Geometry check sheet. Reference: the model listing, model coordinates, mm. Face numbers are marked on the shaded views. A direction names the side the tool comes from. Round coordinates to 2 decimals unless told otherwise and drop trailing zeros. Write each loop counter-clockwise with the first axis right and the second up, starting at its lowest first coordinate (ties: lowest second). Pieces come first, ordered by that corner, then holes. Notation, with made-up numbers: M 30.5,86 L 55.5,86 A17 ccw 55.5,115 Z; hole C 30,21 d5. An arc over 180 degrees is marked long. Use a Markdown table: item, result.
```python
from build123d import *

# Parameters (mm, degrees)
F0_R     = 5
F1_DEPTH = 30
F2_W     = 20
F2_H     = 28
F2_R     = 5
F3_DEPTH = 28
F4_DEPTH = 56
F5_R     = 1
F6_R     = 3
F7_R     = 1


with BuildPart() as f1:
    # F0 (on Front) → F1 (new body)
    with BuildSketch(Plane.XZ):
        Polygon((0, 30), (0, 0), (20, 0), (20, 5), (16, 5), (16, 10), (20, 10), (20, 30), align=None)
        with Locations((10, 20)):
            Circle(F0_R, mode=Mode.SUBTRACT)
    extrude(amount=F1_DEPTH)

    # F2 (on face) → F3 (cut)
    with BuildSketch(Plane.XY.offset(30)):
        with Locations((10, -16)):
            Rectangle(F2_W, F2_H)
        with Locations((10, -20)):
            Circle(F2_R, mode=Mode.SUBTRACT)
        with Locations((10, -20)):
            Circle(F2_R)
    extrude(amount=-F3_DEPTH, mode=Mode.SUBTRACT)

    # F2 (on face) → F4 (cut)
    with BuildSketch(Plane.XY.offset(30)):
        with Locations((10, -20)):
            Circle(F2_R)
    extrude(amount=-F4_DEPTH, mode=Mode.SUBTRACT)

    # F5
    f5_edges = [f1.edges().sort_by_distance(p)[0] for p in [
        (20, -30, 1),
        (0, -30, 1),
        (20, -1, 30),
        (0, -1, 30),
    ]]
    fillet(f5_edges, radius=F5_R)

    # F6
    f6_edges = [f1.edges().sort_by_distance(p)[0] for p in [
        (10, 0, 0),
    ]]
    fillet(f6_edges, radius=F6_R)

    # F7
    f7_edges = [f1.edges().sort_by_distance(p)[0] for p in [
        (10, -2, 2),
    ]]
    fillet(f7_edges, radius=F7_R)


solid = f1.part
```
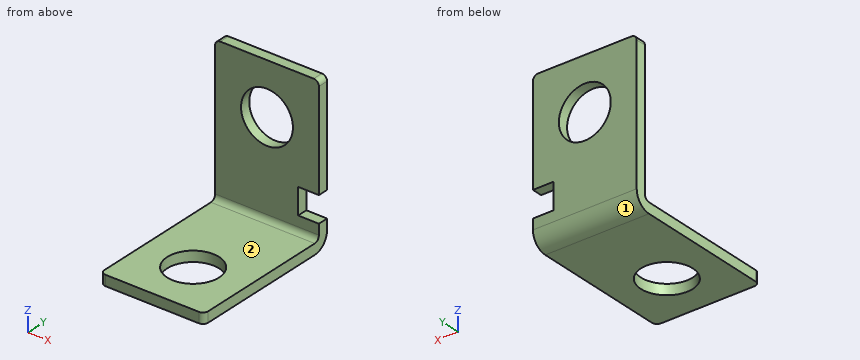
Item 1: Access from +Z, -Z, +X, -X, +Y, -Y to the whole of each face (thin tool, end or side, straight path). Record for the marked faces 1 and 2.
Outcome:
| item | result |
|---|---|
| face 1 | -Z, +X, -X, +Y |
| face 2 | +Z, +X, -X, -Y |
Item 2: Go/stop test with flat-tipped pins: pin 1 (10 mm diameter, centred on x = 9.5, y = -20.5, fed in from +Z); pin 2 (8 mm diameter, centred on y = -6, z = 4.5, fed in from +X); pin 3 (1.6 mm diameter, centred on x = 17, y = -1, fed in from -Z); pin 4 (2 mm diameter, centred on y = -1, z = 8, fed in from +X). Record where each tip stops, or that it passes through.
Outcome:
| item | result |
|---|---|
| pin 1 | stops at z = 2 |
| pin 2 | stops at x = 20 |
| pin 3 | stops at z = 0.25 |
| pin 4 | stops at x = 16 |
Item 3: Cross-section at C-C, the plane z = 20. Record the cut outline in (x, y), and give its area (3 significant figures).
Outcome:
| item | result |
|---|---|
| outline | M 0,-2 L 5,-2 L 5,0 L 0,0 Z; M 15,-2 L 20,-2 L 20,0 L 15,0 Z |
| area | 20.0 mm2 |
Item 4: Cross-section at B-B, the plane y = -20. Record the cut outline in (x, z).
Outcome:
| item | result |
|---|---|
| outline | M 0,0 L 5,0 L 5,2 L 0,2 Z; M 15,0 L 20,0 L 20,2 L 15,2 Z |
Item 5: Cross-section at A-A, the plane x = 10. Record the cut outline in (y, z), and give its area (3 significant figures).
Outcome:
| item | result |
|---|---|
| outline | M -30,0 L -25,0 L -25,2 L -30,2 Z; M -15,0 L -3,0 A3 ccw 0,3 L 0,15 L -2,15 L -2,3 A1 cw -3,2 L -15,2 Z; M -2,25 L 0,25 L 0,30 L -2,30 Z |
| area | 74.3 mm2 |
Item 6: Material ranges on line 1 along X through (y, z) = (-1.5, 20); line 2 along Y through (x, z) = (16, 20.25); line 3 along Z through (x, y) = (4.5, -27.75), recorded low to high. Write a range as from..to.
Outcome:
| item | result |
|---|---|
| line 1 | x = 0..5, 15..20 |
| line 2 | y = -2..0 |
| line 3 | z = 0..2 |
Item 7: Cross-section at D-D, the plane x = 18.5. Record the cut outline in (y, z).
Outcome:
| item | result |
|---|---|
| outline | M -30,0 L -3,0 A3 ccw 0,3 L 0,5 L -2,5 L -2,3 A1 cw -3,2 L -30,2 Z; M -2,10 L 0,10 L 0,30 L -2,30 Z |
